For this review, take the finished solid that the model builds, in its own axes (mm). Round coordinates to 2 decimals unless told otherwise and drop trailing zeros. Write each loop counter-clockwise with the first axis right and the second up, starting at its lowest first coordinate (ties: lowest second). Pieces come first, ordered by that corner, then holes. Notation, with made-up numbers: M -28.75,34 L -3.75,34 A30 ccw -3.75,57 Z; hole C 0.25,64.25 d3. An arc over 180 degrees is marked long. One line per question, with ' | ' between items.
```python
from build123d import *

# Parameters (mm, degrees)
F0_W      = 69.863096
F0_H      = 137.526572
F2_DEPTH  = 76.89179
F1_R      = 9.824635
F4_DEPTH  = 25.4
F4_FACE_W = 69.863096
F4_FACE_H = 137.526572
F5_DEPTH  = 25.4
F6_DEPTH  = 25.4


with BuildPart() as f2:
    # F0 (on Top) → F2 (new body)
    with BuildSketch(Plane.XY):
        with Locations((-34.931548, 0)):
            Rectangle(F0_W, F0_H)
        with Locations((34.931548, 0)):
            Rectangle(F0_W, F0_H)
    extrude(amount=-F2_DEPTH)

    # F1 (on Top) → F3 (revolve)
    with BuildSketch(Plane.XY):
        with Locations((54.264009, 0)):
            Circle(F1_R)
    revolve(axis=Axis((0, 0, 0), (0, -1, 0)))

    # F0 (on Top) → F4 (join)
    with BuildSketch(Plane.XY):
        with Locations((-34.931548, 0)):
            Rectangle(F0_W, F0_H)
    extrude(amount=F4_DEPTH)

    # F4_face (on face) → F5 (join)
    with BuildSketch(Plane(origin=(-34.455236, 0, 25.4), x_dir=(1, 0, 0), z_dir=(0, 0, 1))):
        with Locations((-0.476312, 0)):
            Rectangle(F4_FACE_W, F4_FACE_H)
        with BuildLine():
            add(Edge.make_bspline(
                [(-24.385178, 0), (-24.385178, 0.668247), (-24.32577, 1.336628), (-24.206912, 1.99823), (-24.030098, 2.646689), (-23.797825, 3.276099), (-23.37971, 4.166697), (-23.234065, 4.446908), (-23.077242, 4.721166), (-22.909651, 4.98898), (-22.731734, 5.249905), (-22.229971, 5.927648), (-21.88841, 6.331385), (-21.521456, 6.712873), (-21.131426, 7.070663), (-20.720671, 7.403639), (-19.847998, 8.028648), (-19.384812, 8.318937), (-18.904547, 8.580964), (-18.409705, 8.814186), (-17.902695, 9.018322), (-17.050434, 9.306791), (-16.710914, 9.40802), (-16.367843, 9.496945), (-16.02182, 9.573576), (-15.673419, 9.637946), (-14.585966, 9.79991), (-13.840719, 9.855608), (-13.09247, 9.857734), (-12.345999, 9.807078), (-11.605852, 9.704627), (-10.339404, 9.438416), (-9.80827, 9.297984), (-9.284679, 9.130358), (-8.770428, 8.935906), (-8.267378, 8.715014), (-7.592089, 8.374585), (-7.408591, 8.277395), (-7.227085, 8.176494), (-7.047683, 8.071901), (-6.870499, 7.963641), (-6.45624, 7.69851), (-6.221211, 7.538453), (-5.990868, 7.371624), (-5.765532, 7.198092), (-5.545543, 7.017935), (-5.03891, 6.576543), (-4.757184, 6.309683), (-4.486982, 6.030895), (-4.229294, 5.740472), (-3.985174, 5.4388), (-3.558839, 4.858328), (-3.372758, 4.582367), (-3.198165, 4.298826), (-3.035779, 4.008107), (-2.886315, 3.710707), (-2.67324, 3.234777), (-2.600421, 3.060357), (-2.532119, 2.88409), (-2.468453, 2.706097), (-2.409533, 2.526514), (-2.243048, 1.969131), (-2.15158, 1.586498), (-2.081997, 1.19897), (-2.03498, 0.808045), (-2.01092, 0.415339), (-2.008697, -0.377657), (-2.031422, -0.778015), (-2.078012, -1.17662), (-2.148069, -1.571759), (-2.240876, -1.961843), (-2.409505, -2.526425), (-2.46842, -2.706002), (-2.532082, -2.883988), (-2.600379, -3.060249), (-2.673192, -3.234663), (-2.88625, -3.710575), (-3.035702, -4.007963), (-3.198075, -4.298671), (-3.372655, -4.582202), (-3.55872, -4.858153), (-3.985022, -5.438608), (-4.229123, -5.740271), (-4.486791, -6.030687), (-4.756973, -6.30947), (-5.038678, -6.576325), (-5.545277, -7.017715), (-5.765253, -7.197872), (-5.990575, -7.371405), (-6.220906, -7.538235), (-6.455921, -7.698295), (-6.87016, -7.963432), (-7.047336, -8.071696), (-7.226731, -8.176292), (-7.40823, -8.277198), (-7.591721, -8.374391), (-8.266995, -8.714841), (-8.770037, -8.93575), (-9.284281, -9.130219), (-9.807866, -9.297862), (-10.338996, -9.438312), (-11.605451, -9.704568), (-12.345612, -9.807044), (-13.092098, -9.857724), (-13.840364, -9.85562), (-14.58563, -9.799941), (-15.673115, -9.638001), (-16.021528, -9.573637), (-16.367564, -9.497013), (-16.710646, -9.408093), (-17.050179, -9.306869), (-17.902472, -9.018411), (-18.4095, -8.814279), (-18.90436, -8.58106), (-19.384645, -8.319034), (-19.847849, -8.028745), (-20.720553, -7.403734), (-21.131321, -7.070757), (-21.521364, -6.712964), (-21.888331, -6.331472), (-22.229903, -5.927731), (-22.731682, -5.249979), (-22.909604, -4.989052), (-23.0772, -4.721236), (-23.234028, -4.446976), (-23.379677, -4.166762), (-23.797805, -3.276152), (-24.030086, -2.646733), (-24.206906, -1.998264), (-24.325768, -1.336651), (-24.385178, -0.668258), (-24.385178, 0)],
                knots=[0, 0, 0, 0, 0, 0, 0, 0.060752, 0.060752, 0.060752, 0.060752, 0.060752, 0.089435, 0.089435, 0.089435, 0.089435, 0.089435, 0.137395, 0.137395, 0.137395, 0.137395, 0.137395, 0.186967, 0.186967, 0.186967, 0.186967, 0.186967, 0.219128, 0.219128, 0.219128, 0.219128, 0.219128, 0.286825, 0.286825, 0.286825, 0.286825, 0.286825, 0.336655, 0.336655, 0.336655, 0.336655, 0.336655, 0.355511, 0.355511, 0.355511, 0.355511, 0.355511, 0.381329, 0.381329, 0.381329, 0.381329, 0.381329, 0.416554, 0.416554, 0.416554, 0.416554, 0.416554, 0.446776, 0.446776, 0.446776, 0.446776, 0.446776, 0.463951, 0.463951, 0.463951, 0.463951, 0.463951, 0.499657, 0.499657, 0.499657, 0.499657, 0.499657, 0.536048, 0.536048, 0.536048, 0.536048, 0.536048, 0.553222, 0.553222, 0.553222, 0.553222, 0.553222, 0.583442, 0.583442, 0.583442, 0.583442, 0.583442, 0.618665, 0.618665, 0.618665, 0.618665, 0.618665, 0.644483, 0.644483, 0.644483, 0.644483, 0.644483, 0.663338, 0.663338, 0.663338, 0.663338, 0.663338, 0.713168, 0.713168, 0.713168, 0.713168, 0.713168, 0.780867, 0.780867, 0.780867, 0.780867, 0.780867, 0.813029, 0.813029, 0.813029, 0.813029, 0.813029, 0.862602, 0.862602, 0.862602, 0.862602, 0.862602, 0.910564, 0.910564, 0.910564, 0.910564, 0.910564, 0.939247, 0.939247, 0.939247, 0.939247, 0.939247, 1, 1, 1, 1, 1, 1, 1], degree=6))
        make_face(mode=Mode.SUBTRACT)
    extrude(amount=-F5_DEPTH)

    # F4_face (on face) → F6 (join)
    with BuildSketch(Plane(origin=(-34.455236, 0, 25.4), x_dir=(1, 0, 0), z_dir=(0, 0, 1))):
        with Locations((-0.476312, 0)):
            Rectangle(F4_FACE_W, F4_FACE_H)
        with BuildLine():
            add(Edge.make_bspline(
                [(-24.385178, 0), (-24.385178, 0.668247), (-24.32577, 1.336628), (-24.206912, 1.99823), (-24.030098, 2.646689), (-23.797825, 3.276099), (-23.37971, 4.166697), (-23.234065, 4.446908), (-23.077242, 4.721166), (-22.909651, 4.98898), (-22.731734, 5.249905), (-22.229971, 5.927648), (-21.88841, 6.331385), (-21.521456, 6.712873), (-21.131426, 7.070663), (-20.720671, 7.403639), (-19.847998, 8.028648), (-19.384812, 8.318937), (-18.904547, 8.580964), (-18.409705, 8.814186), (-17.902695, 9.018322), (-17.050434, 9.306791), (-16.710914, 9.40802), (-16.367843, 9.496945), (-16.02182, 9.573576), (-15.673419, 9.637946), (-14.585966, 9.79991), (-13.840719, 9.855608), (-13.09247, 9.857734), (-12.345999, 9.807078), (-11.605852, 9.704627), (-10.339404, 9.438416), (-9.80827, 9.297984), (-9.284679, 9.130358), (-8.770428, 8.935906), (-8.267378, 8.715014), (-7.592089, 8.374585), (-7.408591, 8.277395), (-7.227085, 8.176494), (-7.047683, 8.071901), (-6.870499, 7.963641), (-6.45624, 7.69851), (-6.221211, 7.538453), (-5.990868, 7.371624), (-5.765532, 7.198092), (-5.545543, 7.017935), (-5.03891, 6.576543), (-4.757184, 6.309683), (-4.486982, 6.030895), (-4.229294, 5.740472), (-3.985174, 5.4388), (-3.558839, 4.858328), (-3.372758, 4.582367), (-3.198165, 4.298826), (-3.035779, 4.008107), (-2.886315, 3.710707), (-2.67324, 3.234777), (-2.600421, 3.060357), (-2.532119, 2.88409), (-2.468453, 2.706097), (-2.409533, 2.526514), (-2.243048, 1.969131), (-2.15158, 1.586498), (-2.081997, 1.19897), (-2.03498, 0.808045), (-2.01092, 0.415339), (-2.008697, -0.377657), (-2.031422, -0.778015), (-2.078012, -1.17662), (-2.148069, -1.571759), (-2.240876, -1.961843), (-2.409505, -2.526425), (-2.46842, -2.706002), (-2.532082, -2.883988), (-2.600379, -3.060249), (-2.673192, -3.234663), (-2.88625, -3.710575), (-3.035702, -4.007963), (-3.198075, -4.298671), (-3.372655, -4.582202), (-3.55872, -4.858153), (-3.985022, -5.438608), (-4.229123, -5.740271), (-4.486791, -6.030687), (-4.756973, -6.30947), (-5.038678, -6.576325), (-5.545277, -7.017715), (-5.765253, -7.197872), (-5.990575, -7.371405), (-6.220906, -7.538235), (-6.455921, -7.698295), (-6.87016, -7.963432), (-7.047336, -8.071696), (-7.226731, -8.176292), (-7.40823, -8.277198), (-7.591721, -8.374391), (-8.266995, -8.714841), (-8.770037, -8.93575), (-9.284281, -9.130219), (-9.807866, -9.297862), (-10.338996, -9.438312), (-11.605451, -9.704568), (-12.345612, -9.807044), (-13.092098, -9.857724), (-13.840364, -9.85562), (-14.58563, -9.799941), (-15.673115, -9.638001), (-16.021528, -9.573637), (-16.367564, -9.497013), (-16.710646, -9.408093), (-17.050179, -9.306869), (-17.902472, -9.018411), (-18.4095, -8.814279), (-18.90436, -8.58106), (-19.384645, -8.319034), (-19.847849, -8.028745), (-20.720553, -7.403734), (-21.131321, -7.070757), (-21.521364, -6.712964), (-21.888331, -6.331472), (-22.229903, -5.927731), (-22.731682, -5.249979), (-22.909604, -4.989052), (-23.0772, -4.721236), (-23.234028, -4.446976), (-23.379677, -4.166762), (-23.797805, -3.276152), (-24.030086, -2.646733), (-24.206906, -1.998264), (-24.325768, -1.336651), (-24.385178, -0.668258), (-24.385178, 0)],
                knots=[0, 0, 0, 0, 0, 0, 0, 0.060752, 0.060752, 0.060752, 0.060752, 0.060752, 0.089435, 0.089435, 0.089435, 0.089435, 0.089435, 0.137395, 0.137395, 0.137395, 0.137395, 0.137395, 0.186967, 0.186967, 0.186967, 0.186967, 0.186967, 0.219128, 0.219128, 0.219128, 0.219128, 0.219128, 0.286825, 0.286825, 0.286825, 0.286825, 0.286825, 0.336655, 0.336655, 0.336655, 0.336655, 0.336655, 0.355511, 0.355511, 0.355511, 0.355511, 0.355511, 0.381329, 0.381329, 0.381329, 0.381329, 0.381329, 0.416554, 0.416554, 0.416554, 0.416554, 0.416554, 0.446776, 0.446776, 0.446776, 0.446776, 0.446776, 0.463951, 0.463951, 0.463951, 0.463951, 0.463951, 0.499657, 0.499657, 0.499657, 0.499657, 0.499657, 0.536048, 0.536048, 0.536048, 0.536048, 0.536048, 0.553222, 0.553222, 0.553222, 0.553222, 0.553222, 0.583442, 0.583442, 0.583442, 0.583442, 0.583442, 0.618665, 0.618665, 0.618665, 0.618665, 0.618665, 0.644483, 0.644483, 0.644483, 0.644483, 0.644483, 0.663338, 0.663338, 0.663338, 0.663338, 0.663338, 0.713168, 0.713168, 0.713168, 0.713168, 0.713168, 0.780867, 0.780867, 0.780867, 0.780867, 0.780867, 0.813029, 0.813029, 0.813029, 0.813029, 0.813029, 0.862602, 0.862602, 0.862602, 0.862602, 0.862602, 0.910564, 0.910564, 0.910564, 0.910564, 0.910564, 0.939247, 0.939247, 0.939247, 0.939247, 0.939247, 1, 1, 1, 1, 1, 1, 1], degree=6))
        make_face(mode=Mode.SUBTRACT)
    extrude(amount=-F6_DEPTH)


solid = f2.part
```
Item 1: Take a section at B-B (y = 42.5). Write out the cut boundary in (x, z), then the cut area to 3 significant figures.
Results:
outline: M -69.86,-76.89 L 69.86,-76.89 L 69.86,0 L 0,0 L 0,25.4 L -69.86,25.4 Z | area: 12,500 mm2
Item 2: Take a section at A-A (y = 5). Write out the cut boundary in (x, z), then the cut area to 3 significant figures.
Results:
outline: M -69.86,-76.89 L 69.86,-76.89 L 69.86,0 L 62.72,0 A62.72 ccw -57.35,25.4 L -69.86,25.4 Z; hole M -38.12,25.4 L 0,25.4 L 0,0 L 45.81,0 A45.81 ccw Z | area: 15,000 mm2
Item 3: Insertion check: pin 1 Ø10 at (x, z) = (-32.5, 39) entering from +Y; pin 2 Ø8 at (x, y) = (-39.5, -50) entering from +Z; pin 3 Ø21 at (x, y) = (33.5, 18.5) entering from +Z. Each pin has a flat end and moves straight along its axis. Give the tip position at first contact, or say it passes through.
Results:
pin 1: y = 9.82 | pin 2: z = 25.4 | pin 3: z = 50.85
Item 4: To check wall thickness, follow line 1 along Z through (x, y) = (-9, -45.5); line 2 along Y through (x, z) = (25.5, 48); line 3 along Z through (x, y) = (63.5, 48). State the ranges of each line that lie inside material, in increasing order. Write a range as from..to.
Results:
line 1: -76.89..25.4 | line 2: -9.82..9.82 | line 3: -76.89..0
